Model file for the job. Use its own axes, mm. Face numbers are marked on the shaded views. A direction names the side the tool comes from. Give positions to 0.01 mm unless a question says otherwise; leave off trailing zeros. Loops run counter-clockwise (first coordinate to the right, second up) from the corner with the lowest first, then second, coordinate; pieces in that order, holes last. Notation, with made-up numbers: (87, -24.75) - (91, -24.75) arc R20 cw to (91, 3.25) - close; hole circle Ø9 at (32, -24.75). An arc over 180 degrees is marked (long way). Answer as CSV lines item,"result". Start each with the question number.
Item 1: Pin check, flat tips, straight feed: pin 1 (1.5 mm diameter, centred on x = -4, y = -6.5, fed in from +Z); pin 2 (5.5 mm diameter, centred on x = 3.31, y = -5.52, fed in from +Z); pin 3 (5.5 mm diameter, centred on x = 3.28, y = -5.52, fed in from -Z). Stop position of each tip, or through.
Item 2: Drill centre lines: L1, parallel to X at y = -7, z = -0.5; L2, parallel to X at y = -13.75, z = -0.4; L3, parallel to X at y = 0.5, z = -0.35. Where is each one in solid material? Low to high. Write a range as from..to.
Item 3: Tool access for the marked faces 1 and 2: list every direction of +Z, -Z, +X, -X, +Y, -Y with a clear straight run to the whole face (end or side of a thin tool).
Item 4: Saw through at C-C on x = -25. Give the cut face in (y, z), plus the area to 3 significant figures.
Item 5: Saw through at B-B on y = 2.5. Give the cut face in (x, z).
Item 6: Saw through at A-A on y = -6.25. Give the cut face in (x, z), plus the area to 3 significant figures.
from build123d import *

# Parameters (mm, degrees)
F1_DEPTH  = 2.1
F2_R      = 1.5
F3_DEPTH  = 2.101
F5_DEPTH  = 0.8
F6_R      = 4.5
F6_R_2    = 1.5
F7_DEPTH  = 0.8
F9_DEPTH  = 20
F10_R     = 0.75
F11_DEPTH = 20.001


# Not quite as in the source:
# - a feature names something its author has since deleted; it is built from what else it names


with BuildPart() as f1:
    # F0 (on Top) → F1 (new body)
    with BuildSketch(Plane.XY):
        with BuildLine():
            Line((-61.724215433, 4.4804378226), (-61.724215433, -15.5195621774))
            Line((-61.724215433, -15.5195621774), (10.275784567, -15.5195621774))
            ThreePointArc((10.275784567, -15.5195621774), (13.1042116917, -14.3479893021), (14.275784567, -11.5195621774))
            Line((14.275784567, -11.5195621774), (14.275784567, -5.5195621774))
            Line((14.275784567, -5.5195621774), (14.275784567, 0.4804378226))
            ThreePointArc((14.275784567, 0.4804378226), (13.1042116917, 3.3088649474), (10.275784567, 4.4804378226))
            Line((10.275784567, 4.4804378226), (-61.724215433, 4.4804378226))
        make_face()
    extrude(amount=-F1_DEPTH)

    # F2 (on face) → F3 (cut, through all)
    with BuildSketch(Plane(origin=(0, 0, -2.1), x_dir=(1, 0, 0), z_dir=(0, 0, -1))):
        with Locations((3.2757834997, 5.5195621774)):
            Circle(F2_R)
    extrude(amount=-F3_DEPTH, mode=Mode.SUBTRACT)

    # F4 (on face) → F5 (cut)
    with BuildSketch(Plane.XY):
        with BuildLine():
            ThreePointArc((6.808292926, -5.5195621774), (-0.1917041784, -5.5256023727), (6.8082952425, -5.523588974))
            ThreePointArc((6.8082952425, -5.523588974), (6.8082946634, -5.5215755754), (6.808292926, -5.5195621774))
        make_face()
    extrude(amount=-F5_DEPTH, mode=Mode.SUBTRACT)

    # F6 (on face) → F7 (cut)
    with BuildSketch(Plane(origin=(0, 0, -2.1), x_dir=(1, 0, 0), z_dir=(0, 0, -1))):
        with Locations((3.2757834997, 5.5195621774)):
            Circle(F6_R)
        with Locations((3.2757834997, 5.5195621774)):
            Circle(F6_R_2, mode=Mode.SUBTRACT)
    extrude(amount=-F7_DEPTH, mode=Mode.SUBTRACT)

    # F8 (on face) → F9 (join)
    with BuildSketch(Plane.XZ.offset(15.5195621774)):
        with BuildLine():
            Line((-59.1665172217, 2.5), (-61.724215433, 2.5))
            Line((-61.724215433, 2.5), (-61.724215433, 0))
            Line((-61.724215433, 0), (-57.1891452284, 0))
            Line((-57.1891452284, 0), (-56.3891452284, 0))
            ThreePointArc((-56.3891452284, 0), (-56.9548306533, 0.2343145751), (-57.1891452284, 0.8))
            ThreePointArc((-57.1891452284, 0.8), (-57.8626767407, 2.0165750888), (-59.1665172217, 2.5))
        make_face()
    extrude(amount=-F9_DEPTH)

    # F10 (on face) → F11 (cut, through all)
    with BuildSketch(Plane(origin=(0, 4.4804378226, 0), x_dir=(-1, 0, 0), z_dir=(0, 1, 0))):
        with Locations((59.05039973, 0.0338958319)):
            Circle(F10_R)
    extrude(amount=-F11_DEPTH, mode=Mode.SUBTRACT)


solid = f1.part
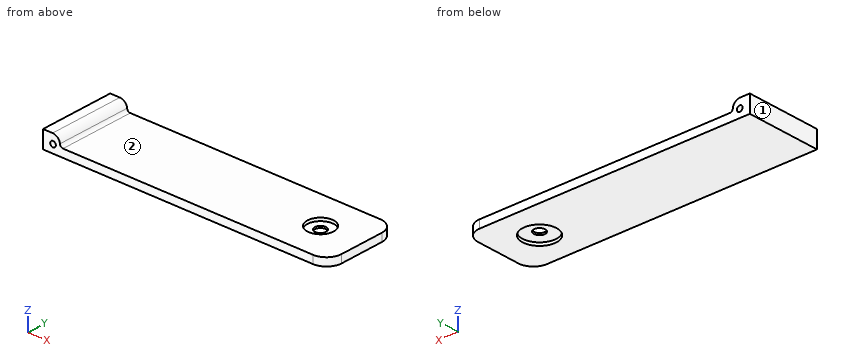
Responses:
1,pin 1,"z = 0"
1,pin 2,"z = -0.8"
1,pin 3,"z = -1.3"
2,L1,"-61.72..-59.58, -58.52..0.13, 6.48..14.28"
2,L2,"-61.72..-59.66, -58.44..13.6"
2,L3,"-61.72..-59.69, -58.41..14.28"
3,face 1,"+Z, -Z, -X, +Y, -Y"
3,face 2,"+Z, +X, +Y, -Y"
4,outline,"(-15.52, -2.1) - (4.48, -2.1) - (4.48, 0) - (-15.52, 0) - close"
4,area,"42.0 mm2"
5,outline,"(-61.72, -2.1) - (13.73, -2.1) - (13.73, 0) - (-56.39, 0) arc R0.8 cw to (-57.19, 0.8) arc R2 ccw to (-59.17, 2.5) - (-61.72, 2.5) - close; hole circle Ø1.5 at (-59.05, 0.03)"
6,outline,"(-61.72, -2.1) - (-1.16, -2.1) - (-1.16, -1.3) - (1.97, -1.3) - (1.97, -0.8) - (-0.12, -0.8) - (-0.12, 0) - (-56.39, 0) arc R0.8 cw to (-57.19, 0.8) arc R2 ccw to (-59.17, 2.5) - (-61.72, 2.5) - close; (4.59, -1.3) - (7.72, -1.3) - (7.72, -2.1) - (14.28, -2.1) - (14.28, 0) - (6.73, 0) - (6.73, -0.8) - (4.59, -0.8) - close; hole circle Ø1.5 at (-59.05, 0.03)"
6,area,"155 mm2"
